Work out the finished part from the listing and answer in its coordinate system (mm). Coordinates: 2 decimals unless noted, no trailing zeros. Write each loop counter-clockwise with the first axis right and the second up, starting at its lowest first coordinate (ties: lowest second). Pieces come first, ordered by that corner, then holes. Notation, with made-up numbers: (16.5, 22.25) - (43.5, 22.25) arc R17 ccw to (43.5, 46.25) - close; hole circle Ø7 at (37, -37). An arc over 180 degrees is marked (long way). Use a Markdown table: item, result. Add a question column.
(1) The part is cut by section A-A, the plane y = 8.25. State how many separate pieces and enclosed holes the cut face has, then the cut area to 3 significant figures.
(2) Find the intervals of material crossed by line 1 (X direction, y = 5.75, z = 60); line 2 (Z direction, x = -78, y = 8.25); line 3 (X direction, y = 3.75, z = -104), in increasing order. Write a range as from..to.
(3) Given pin 1 Ø13 at (x, z) = (-54.28, 39.81) entering from +Y; pin 2 Ø25 at (x, z) = (-54.28, 62.76) entering from +Y, each flat-ended and moving along its own axis, determine where each tip first touches the part or whether it passes through.
(4) The part is cut by section C-C, the plane z = -100. Give the vertices of the cut face in (x, y), then the cut area to 3 significant figures.
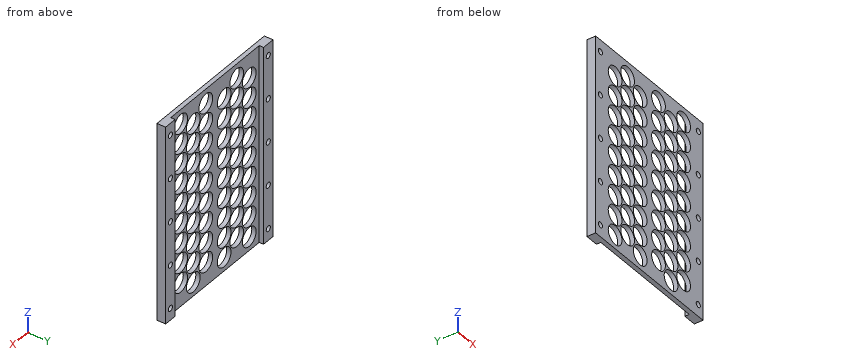
from build123d import *

# Parameters (mm, degrees)
CELL_BLOCK_SKETCH_W  = 140.101132068
CELL_BLOCK_SKETCH_H  = 227.325
BOSS_EXTRUDE1_DEPTH  = 5
CELL_HOLES_PATTERN_R = 10.875
CUT_EXTRUDE1_DEPTH   = 5
SKETCH1_R            = 10.875
CUT_EXTRUDE2_DEPTH   = 5
SKETCH3_W            = 15
SKETCH3_H            = 227.325
BOSS_EXTRUDE3_DEPTH  = 10
SKETCH4_R            = 3.25
CUT_EXTRUDE3_DEPTH   = 10


with BuildPart() as part:
    # Cell Block Sketch → Boss-Extrude1 (new body)
    with BuildSketch(Plane(origin=(0, 0, 0), x_dir=(1, 0, 0), z_dir=(0, 1, 0))):
        Rectangle(CELL_BLOCK_SKETCH_W, CELL_BLOCK_SKETCH_H)
    extrude(amount=BOSS_EXTRUDE1_DEPTH)

    # Cell Holes Pattern → Cut-Extrude1 (cut)
    with BuildSketch(Plane(origin=(0, 0, 0), x_dir=(1, 0, 0), z_dir=(0, 1, 0))):
        with Locations(Location((-34.400283017, 86.4125, 0), (0, 0, 270))):
            Circle(CELL_HOLES_PATTERN_R)
        with Locations(Location((-54.275566034, 97.8875, 0), (0, 0, 270))):
            Circle(CELL_HOLES_PATTERN_R)
        with Locations(Location((-14.525, 97.8875, 0), (0, 0, 270))):
            Circle(CELL_HOLES_PATTERN_R)
        with Locations(Location((-54.275566034, 74.9375, 0), (0, 0, 270))):
            Circle(CELL_HOLES_PATTERN_R)
        with Locations(Location((-34.400283017, 63.4625, 0), (0, 0, 270))):
            Circle(CELL_HOLES_PATTERN_R)
        with Locations(Location((-14.525, 74.9375, 0), (0, 0, 270))):
            Circle(CELL_HOLES_PATTERN_R)
        with Locations(Location((-54.275566034, 51.9875, 0), (0, 0, 270))):
            Circle(CELL_HOLES_PATTERN_R)
        with Locations(Location((-34.400283017, 40.5125, 0), (0, 0, 270))):
            Circle(CELL_HOLES_PATTERN_R)
        with Locations(Location((-14.525, 51.9875, 0), (0, 0, 270))):
            Circle(CELL_HOLES_PATTERN_R)
        with Locations(Location((-54.275566034, 29.0375, 0), (0, 0, 270))):
            Circle(CELL_HOLES_PATTERN_R)
        with Locations(Location((-34.400283017, 17.5625, 0), (0, 0, 270))):
            Circle(CELL_HOLES_PATTERN_R)
        with Locations(Location((-14.525, 29.0375, 0), (0, 0, 270))):
            Circle(CELL_HOLES_PATTERN_R)
        with Locations(Location((-54.275566034, 6.0875, 0), (0, 0, 270))):
            Circle(CELL_HOLES_PATTERN_R)
        with Locations(Location((-34.400283017, -5.3875, 0), (0, 0, 270))):
            Circle(CELL_HOLES_PATTERN_R)
        with Locations(Location((-14.525, 6.0875, 0), (0, 0, 270))):
            Circle(CELL_HOLES_PATTERN_R)
        with Locations(Location((-54.275566034, -16.8625, 0), (0, 0, 270))):
            Circle(CELL_HOLES_PATTERN_R)
        with Locations(Location((-34.400283017, -28.3375, 0), (0, 0, 270))):
            Circle(CELL_HOLES_PATTERN_R)
        with Locations(Location((-14.525, -16.8625, 0), (0, 0, 270))):
            Circle(CELL_HOLES_PATTERN_R)
        with Locations(Location((-54.275566034, -39.8125, 0), (0, 0, 270))):
            Circle(CELL_HOLES_PATTERN_R)
        with Locations(Location((-34.400283017, -51.2875, 0), (0, 0, 270))):
            Circle(CELL_HOLES_PATTERN_R)
        with Locations(Location((-14.525, -39.8125, 0), (0, 0, 270))):
            Circle(CELL_HOLES_PATTERN_R)
        with Locations(Location((-54.275566034, -62.7625, 0), (0, 0, 270))):
            Circle(CELL_HOLES_PATTERN_R)
        with Locations(Location((-34.400283017, -74.2375, 0), (0, 0, 270))):
            Circle(CELL_HOLES_PATTERN_R)
        with Locations(Location((-14.525, -62.7625, 0), (0, 0, 270))):
            Circle(CELL_HOLES_PATTERN_R)
        with Locations(Location((-54.275566034, -85.7125, 0), (0, 0, 270))):
            Circle(CELL_HOLES_PATTERN_R)
        with Locations(Location((-34.400283017, -97.1875, 0), (0, 0, 270))):
            Circle(CELL_HOLES_PATTERN_R)
        with Locations(Location((-14.525, -85.7125, 0), (0, 0, 270))):
            Circle(CELL_HOLES_PATTERN_R)
    extrude(amount=CUT_EXTRUDE1_DEPTH, mode=Mode.SUBTRACT)

    # Sketch1 → Cut-Extrude2 (cut)
    with BuildSketch(Plane(origin=(0, 5, 0), x_dir=(1, 0, 0), z_dir=(0, 1, 0))):
        with Locations(Location((14.525, 86.4125, 0), (0, 0, 270))):
            Circle(SKETCH1_R)
        with Locations(Location((34.400283017, 97.8875, 0), (0, 0, 270))):
            Circle(SKETCH1_R)
        with Locations(Location((54.275566034, 86.4125, 0), (0, 0, 270))):
            Circle(SKETCH1_R)
        with Locations(Location((14.525, 63.4625, 0), (0, 0, 270))):
            Circle(SKETCH1_R)
        with Locations(Location((34.400283017, 74.9375, 0), (0, 0, 270))):
            Circle(SKETCH1_R)
        with Locations(Location((54.275566034, 63.4625, 0), (0, 0, 270))):
            Circle(SKETCH1_R)
        with Locations(Location((14.525, 40.5125, 0), (0, 0, 270))):
            Circle(SKETCH1_R)
        with Locations(Location((34.400283017, 51.9875, 0), (0, 0, 270))):
            Circle(SKETCH1_R)
        with Locations(Location((54.275566034, 40.5125, 0), (0, 0, 270))):
            Circle(SKETCH1_R)
        with Locations(Location((14.525, 17.5625, 0), (0, 0, 270))):
            Circle(SKETCH1_R)
        with Locations(Location((34.400283017, 29.0375, 0), (0, 0, 270))):
            Circle(SKETCH1_R)
        with Locations(Location((54.275566034, 17.5625, 0), (0, 0, 270))):
            Circle(SKETCH1_R)
        with Locations(Location((14.525, -5.3875, 0), (0, 0, 270))):
            Circle(SKETCH1_R)
        with Locations(Location((34.400283017, 6.0875, 0), (0, 0, 270))):
            Circle(SKETCH1_R)
        with Locations(Location((54.275566034, -5.3875, 0), (0, 0, 270))):
            Circle(SKETCH1_R)
        with Locations(Location((14.525, -28.3375, 0), (0, 0, 270))):
            Circle(SKETCH1_R)
        with Locations(Location((34.400283017, -16.8625, 0), (0, 0, 270))):
            Circle(SKETCH1_R)
        with Locations(Location((54.275566034, -28.3375, 0), (0, 0, 270))):
            Circle(SKETCH1_R)
        with Locations(Location((14.525, -51.2875, 0), (0, 0, 270))):
            Circle(SKETCH1_R)
        with Locations(Location((34.400283017, -39.8125, 0), (0, 0, 270))):
            Circle(SKETCH1_R)
        with Locations(Location((54.275566034, -51.2875, 0), (0, 0, 270))):
            Circle(SKETCH1_R)
        with Locations(Location((14.525, -74.2375, 0), (0, 0, 270))):
            Circle(SKETCH1_R)
        with Locations(Location((34.400283017, -62.7625, 0), (0, 0, 270))):
            Circle(SKETCH1_R)
        with Locations(Location((54.275566034, -74.2375, 0), (0, 0, 270))):
            Circle(SKETCH1_R)
        with Locations(Location((14.525, -97.1875, 0), (0, 0, 270))):
            Circle(SKETCH1_R)
        with Locations(Location((34.400283017, -85.7125, 0), (0, 0, 270))):
            Circle(SKETCH1_R)
        with Locations(Location((54.275566034, -97.1875, 0), (0, 0, 270))):
            Circle(SKETCH1_R)
    extrude(amount=-CUT_EXTRUDE2_DEPTH, mode=Mode.SUBTRACT)

    # Sketch3 → Boss-Extrude3 (add)
    with BuildSketch(Plane(origin=(0, 0, 0), x_dir=(1, 0, 0), z_dir=(0, 1, 0))):
        with Locations((-77.550566034, 0)):
            Rectangle(SKETCH3_W, SKETCH3_H)
    boss_extrude3 = extrude(amount=BOSS_EXTRUDE3_DEPTH)

    # Mirror1: Boss-Extrude3 across plane
    add(boss_extrude3.mirror(Plane(origin=(0, 0, 0), x_dir=(0, 0, 1), z_dir=(1, 0, 0))))

    # Sketch4 → Cut-Extrude3 (cut)
    with BuildSketch(Plane(origin=(0, 10, 0), x_dir=(1, 0, 0), z_dir=(0, 1, 0))):
        with Locations(Location((-77.550566034, 0, 0), (0, 0, 270))):
            Circle(SKETCH4_R)
        with Locations(Location((-77.550566034, -50, 0), (0, 0, 270))):
            Circle(SKETCH4_R)
        with Locations(Location((-77.550566034, -100, 0), (0, 0, 270))):
            Circle(SKETCH4_R)
        with Locations(Location((-77.550566034, 50, 0), (0, 0, 270))):
            Circle(SKETCH4_R)
        with Locations(Location((-77.550566034, 100, 0), (0, 0, 270))):
            Circle(SKETCH4_R)
    cut_extrude3 = extrude(amount=-CUT_EXTRUDE3_DEPTH, mode=Mode.SUBTRACT)

    # Mirror2: Cut-Extrude3 across plane
    add(cut_extrude3.mirror(Plane(origin=(0, 0, 0), x_dir=(0, 0, 1), z_dir=(1, 0, 0))), mode=Mode.SUBTRACT)


solid = part.part
Model answer:
| question | item | result |
|---|---|---|
| 1 | separate pieces | 2 |
| 1 | enclosed holes | 10 |
| 1 | area | 6,490 mm^2 |
| 2 | line 1 | -85.05..-70.05, 70.05..85.05 |
| 2 | line 2 | -113.66..-103.22, -96.78..-53.22, -46.78..-3.22, 3.22..46.78, 53.22..96.78, 103.22..113.66 |
| 2 | line 3 | -85.05..-63.27, -45.28..-23.52, -5.53..25.41, 43.39..85.05 |
| 3 | pin 1 | through |
| 3 | pin 2 | y = 5 |
| 4 | outline | (-85.05, 0) - (-80.8, 0) - (-80.8, 10) - (-85.05, 10) - close; (-74.3, 0) - (-64.94, 0) - (-64.94, 5) - (-70.05, 5) - (-70.05, 10) - (-74.3, 10) - close; (-43.61, 0) - (-25.19, 0) - (-25.19, 5) - (-43.61, 5) - close; (-3.86, 0) - (23.73, 0) - (23.73, 5) - (-3.86, 5) - close; (45.07, 0) - (74.3, 0) - (74.3, 10) - (70.05, 10) - (70.05, 5) - (45.07, 5) - close; (80.8, 0) - (85.05, 0) - (85.05, 10) - (80.8, 10) - close |
| 4 | area | 550 mm^2 |
